from build123d import *

# Parameters (mm, degrees)
F0_R     = 25.4
F1_DEPTH = 25.4
F2_W     = 12.7
F2_H     = 76.2
F3_DEPTH = 43.18
F4_R     = 6.35
F4_W     = 19.05
F4_H     = 17.78
F5_DEPTH = 25.4


with BuildPart() as f1:
    # F0 (on Top) → F1 (new body, symmetric)
    with BuildSketch(Plane.XY):
        Circle(F0_R)
    extrude(amount=F1_DEPTH, both=True)

    # F2 (on face) → F3 (cut)
    with BuildSketch(Plane.XY.offset(25.4)):
        Rectangle(F2_W, F2_H)
        with Locations((25.4, 0)):
            Rectangle(F2_W, F2_H)
        with Locations((-25.4, 0)):
            Rectangle(F2_W, F2_H)
    extrude(amount=-F3_DEPTH, mode=Mode.SUBTRACT)

    # F4 (on Right) → F5 (cut, symmetric)
    with BuildSketch(Plane.YZ):
        Circle(F4_R)
        with BuildLine():
            ThreePointArc((-19.05, 0), (0, 19.05), (19.05, 0))
            Line((19.05, 0), (38.1, 0))
            Line((38.1, 0), (38.1, 38.1))
            Line((38.1, 38.1), (-38.1, 38.1))
            Line((-38.1, 38.1), (-38.1, 0))
            Line((-38.1, 0), (-19.05, 0))
        make_face()
        with Locations((28.575, -8.89)):
            Rectangle(F4_W, F4_H)
        with Locations((-28.575, -8.89)):
            Rectangle(F4_W, F4_H)
    extrude(amount=F5_DEPTH, both=True, mode=Mode.SUBTRACT)


solid = f1.part
Input: part model. Units: mm. Frame: model coordinates. A direction names the side the tool comes from. Coordinates: 2 decimals unless noted, no trailing zeros. Loops run counter-clockwise (first coordinate to the right, second up) from the corner with the lowest first, then second, coordinate; pieces in that order, holes last. Notation, with made-up numbers: (43.25, -29.5) -> (99.25, -29.5) arc R10 cw to (99.25, -15.5) -> close; hole circle Ø6 at (4, 89). An arc over 180 degrees is marked (long way). Write each question's results on one line, items separated by ' | '. Start each with the question number.
Q1. Section B-B, the plane y = 0. Return the cut outline in (x, z), plus the area to 4 significant figures.
Q2. Reachability of faces 1 (the flat face through (-12, 19.05, -9)), 2 (the flat face through (-6.35, 0, -7)), 3 (the flat face through (21, 0, -17.78)), 4 (the flat face through (12, -19.05, -9)) from +Z, -Z, +X, -X, +Y, -Y: full face, straight path, thin tool, end or side. Return the list, or none.
Q3. Section D-D, the plane z = 4.5. Return the cut outline in (x, y), plus the area to 3 significant figures.
Q4. Pull-direction query (Y, two-part tool) for faces 5 (the cylindrical face through (12.61, -1.38, -6.2)), 6 (the cylindrical face through (25.27, 2.58, -19.59)), 7 (the flat face through (-22, 0, -17.78)); classes: released by +Y, released by -Y, zero draft, split by the parting line, or undercut.
Q5. Ray query, line 1 (X direction, y = -3.5, z = 15.5); line 2 (Z direction, x = 15, y = 0). Return the intervals inside material, ascending. Write a range as from..to.
Q6. Section C-C, the plane x = 7.5. Return the cut outline in (y, z).
Q7. Pin query (flat end, axial travel): pin 1 (14.5 mm diameter, centred on y = 0, z = 0, fed in from -X); pin 2 (5 mm diameter, centred on x = -23, y = 1.5, fed in from +Z); pin 3 (1.5 mm diameter, centred on x = 9, z = -6, fed in from -Y). Return the tip coordinate at first contact, or that it passes through.
Q8. Section A-A, the plane z = -10.5. Return the cut outline in (x, y), plus the area to 3 significant figures.
Found:
1) outline: (-25.4, -25.4) -> (25.4, -25.4) -> (25.4, -17.78) -> (19.05, -17.78) -> (19.05, -6.35) -> (6.35, -6.35) -> (6.35, -17.78) -> (-6.35, -17.78) -> (-6.35, -6.35) -> (-19.05, -6.35) -> (-19.05, -17.78) -> (-25.4, -17.78) -> close; (-19.05, 6.35) -> (-6.35, 6.35) -> (-6.35, 19.05) -> (-19.05, 19.05) -> close; (6.35, 6.35) -> (19.05, 6.35) -> (19.05, 19.05) -> (6.35, 19.05) -> close | area: 1,000 mm2
2) face 1: +Z, +X, -X, +Y | face 2: +Z, +Y, -Y | face 3: +Z, +X, +Y, -Y | face 4: +Z, +X, -X, -Y
3) outline: (-19.05, -16.8) arc R25.4 ccw to (-17.39, -18.51) -> (-6.35, -18.51) -> (-6.35, -4.48) -> (-19.05, -4.48) -> close; (-19.05, 4.48) -> (-6.35, 4.48) -> (-6.35, 18.51) -> (-17.39, 18.51) arc R25.4 ccw to (-19.05, 16.8) -> close; (6.35, -18.51) -> (17.39, -18.51) arc R25.4 ccw to (19.05, -16.8) -> (19.05, -4.48) -> (6.35, -4.48) -> close; (6.35, 4.48) -> (19.05, 4.48) -> (19.05, 16.8) arc R25.4 ccw to (17.39, 18.51) -> (6.35, 18.51) -> close | area: 707 mm2
4) face 5: undercut | face 6: split by the parting line | face 7: zero draft
5) line 1: -19.05..-6.35, 6.35..19.05 | line 2: -25.4..-6.35, 6.35..19.05
6) outline: (-24.27, -25.4) -> (24.27, -25.4) -> (24.27, -17.78) -> (19.05, -17.78) -> (19.05, 0) arc R19.05 ccw to (-19.05, 0) -> (-19.05, -17.78) -> (-24.27, -17.78) -> close; hole circle Ø12.7 at (0, 0)
7) pin 1: x = -19.05 | pin 2: z = -17.78 | pin 3: y = -19.05
8) outline: (-19.05, -16.8) arc R25.4 ccw to (-16.8, -19.05) -> (-6.35, -19.05) -> (-6.35, 19.05) -> (-16.8, 19.05) arc R25.4 ccw to (-19.05, 16.8) -> close; (6.35, -19.05) -> (16.8, -19.05) arc R25.4 ccw to (19.05, -16.8) -> (19.05, 16.8) arc R25.4 ccw to (16.8, 19.05) -> (6.35, 19.05) -> close | area: 958 mm2
